```python
from build123d import *

# Parameters (mm, degrees)
SKETCH_1_R          = 40
EXTRUDE_1_DEPTH     = 10
SKETCH_2_R          = 38.5
CUT_EXTRUDE_1_DEPTH = 7
SKETCH_4_R          = 1.5
CUT_EXTRUDE_2_DEPTH = 58.445626465


with BuildPart() as part:
    # 草图1 → 凸台-拉伸1 (new body)
    with BuildSketch(Plane.XY):
        Circle(SKETCH_1_R)
    extrude(amount=EXTRUDE_1_DEPTH)

    # 草图2 → 切除-拉伸1 (cut)
    with BuildSketch(Plane(origin=(0, 0, 0), x_dir=(-1, 0, 0), z_dir=(0, 0, -1))):
        Circle(SKETCH_2_R)
    extrude(amount=-CUT_EXTRUDE_1_DEPTH, mode=Mode.SUBTRACT)

    # 草图4 → 切除-拉伸2 (cut, through all)
    with BuildSketch(Plane.XY.offset(10)):
        with Locations((0, 17.67766953)):
            Circle(SKETCH_4_R)
        with Locations((17.67766953, 0)):
            Circle(SKETCH_4_R)
        with Locations((0, -17.67766953)):
            Circle(SKETCH_4_R)
        with Locations((-17.67766953, 0)):
            Circle(SKETCH_4_R)
        Circle(SKETCH_4_R)
    extrude(amount=-CUT_EXTRUDE_2_DEPTH, mode=Mode.SUBTRACT)


solid = part.part
```
The model under review builds one solid part; all positions refer to its coordinate system, in mm. A direction names the side the tool comes from. Coordinates: 2 decimals unless noted, no trailing zeros. Write each loop counter-clockwise with the first axis right and the second up, starting at its lowest first coordinate (ties: lowest second). Pieces come first, ordered by that corner, then holes. Notation, with made-up numbers: (19, 46) -> (29, 46) arc R16 cw to (29, 71) -> close; hole circle Ø5 at (6.5, 77). An arc over 180 degrees is marked (long way). One line per item, written item: value. Start each with the question number.
Q1. For faces 1 (the face through (30.55, -23.43, 3.45)), 2 (the face through (-1.5, 0.07, 8.52)), list the 3-axis set-ups (+Z, -Z, +X, -X, +Y, -Y) from which the entire face can be reached by the end or side of a thin tool; tool diameter is ignored.
Q2. Clearance check with flat-ended pins moving along their axes: P1, Ø4, axis at y = -17, z = 4, coming from the -X side; P2, Ø1, axis at x = -26, z = 7, coming from the +Y side; P3, Ø3, axis at y = -27.5, z = 8, coming from the +X side. State where each tip first meets the part, or that it passes through.
Q3. Add section C-C, the plane y = 33. Give the boundary of the cut face in (x, z), then the cut area to 3 significant figures.
Q4. To check wall thickness, follow probe 1 along Y at (x, z) = (0, 4); probe 2 along Z at (x, y) = (-19, 3); probe 3 along Y at (x, z) = (17, 5.5). State the ranges of each line that lie inside material, in increasing order.
Q5. Add section A-A, the plane x = 0. Give the boundary of the cut face in (y, z).
Q6. Add section D-D, the plane z = 3.5. Give the boundary of the cut face in (x, y).
Q7. The part is to be moulded in two halves that separate along X. For faces 3 (the face through (16.18, 0.07, 8.52)), 4 (the face through (-21, 33, 0)), 5 (the face through (-8.67, -39.05, 4.93)), say which applies: +X half, -X half, draft (parallel to the pull), parting line (faces both ways), or undercut.
Response:
1. face 1: -Z
1. face 2: +Z, -Z
2. P1: x = -37.08
2. P2: y = 30.82
2. P3: x = 30.4
3. outline: (-22.61, 0) -> (-19.83, 0) -> (-19.83, 7) -> (19.83, 7) -> (19.83, 0) -> (22.61, 0) -> (22.61, 10) -> (-22.61, 10) -> close
3. area: 174 mm²
4. probe 1: -40 to -38.5, 38.5 to 40
4. probe 2: 7 to 10
4. probe 3: -36.21 to -34.54, 34.54 to 36.21
5. outline: (-40, 0) -> (-38.5, 0) -> (-38.5, 7) -> (-19.18, 7) -> (-19.18, 10) -> (-40, 10) -> close; (-16.18, 7) -> (-1.5, 7) -> (-1.5, 10) -> (-16.18, 10) -> close; (1.5, 7) -> (16.18, 7) -> (16.18, 10) -> (1.5, 10) -> close; (19.18, 7) -> (38.5, 7) -> (38.5, 0) -> (40, 0) -> (40, 10) -> (19.18, 10) -> close
6. outline: circle Ø80 at (0, 0); hole circle Ø77 at (0, 0)
7. face 3: undercut
7. face 4: draft
7. face 5: parting line
